Input: part model. Units: mm. Frame: model coordinates. Coordinates: 2 decimals unless noted, no trailing zeros. Loops run counter-clockwise (first coordinate to the right, second up) from the corner with the lowest first, then second, coordinate; pieces in that order, holes last. Notation, with made-up numbers: M -13.75,9.25 L 38.25,9.25 A21 cw 38.25,20.25 Z; hole C -25.5,-3 d2. An arc over 180 degrees is marked long. Use a Markdown table: item, result. Add a question column.
1. Line query: L1, parallel to Z at x = 0.95, y = 52.5 (3 decimals); L2, parallel to Y at x = 3.2, z = -154.5; L3, parallel to Z at x = 3.5, y = 17.5 (3 decimals). Output: solid intervals per line, ascending. Write a range as [from, to].
2. Section C-C on z = -126. Output: boundary loops of the cut face in (x, y).
3. Section A-A on x = 3.05. Output: boundary loops of the cut face in (y, z).
4. Pin query (flat end, axial travel): pin 1 (1.5 mm diameter, centred on y = 64.5, z = -147, fed in from +X); pin 2 (1.5 mm diameter, centred on x = 3.5, z = -185, fed in from +Y). Return the tip coordinate at first contact, or that it passes through.
5. Section B-B on y = 107. Output: boundary loops of the cut face in (x, z).
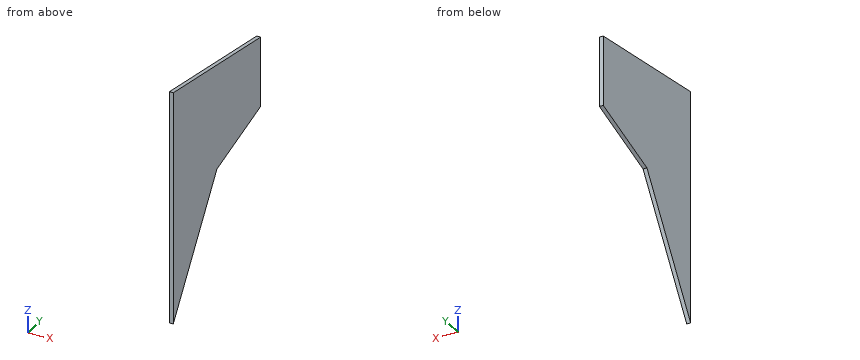
```python
from build123d import *

# Parameters (mm, degrees)
EXTRUDE_2_DEPTH = 5


with BuildPart() as part:
    # 草图1 → 拉伸2 (new body)
    with BuildSketch(Plane(origin=(0, 0, 0), x_dir=(0, 0, -1), z_dir=(1, 0, 0))):
        Polygon((-30, 200), (-60, 0), (120, 0), (90, 100), (60, 200), align=None)
        Polygon((90, 100), (120, 0), (240, 0), align=None)
    extrude(amount=EXTRUDE_2_DEPTH)


solid = part.part
```
Answers below:
| question | item | result |
|---|---|---|
| 1 | L1 | z = [-161.25, 52.125] |
| 1 | L2 | y = [0, 57] |
| 1 | L3 | z = [-213.75, 57.375] |
| 2 | outline | M 0,0 L 5,0 L 5,76 L 0,76 Z |
| 3 | outline | M 0,-240 L 100,-90 L 200,-60 L 200,30 L 0,60 Z |
| 4 | pin 1 | passes through |
| 4 | pin 2 | stops at y = 37.17 |
| 5 | outline | M 0,-87.9 L 5,-87.9 L 5,43.95 L 0,43.95 Z |
